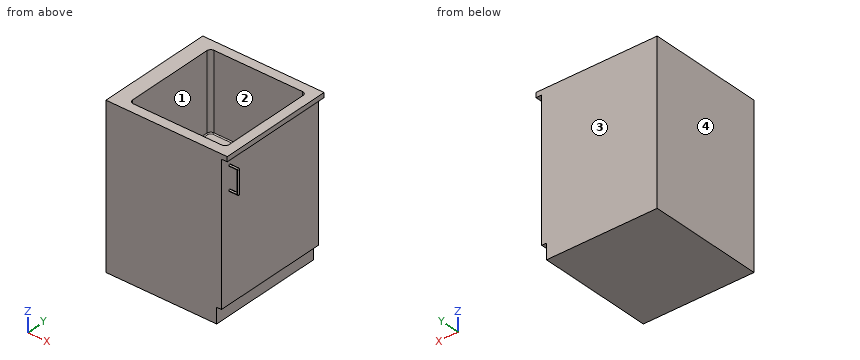
```python
from build123d import *

# Parameters (mm, degrees)
F0_W        = 600
F0_H        = 600
F1_DEPTH    = 800
F2_W        = 600
F2_H        = 80
F3_DEPTH    = 25
F5_DEPTH    = 50
F6_T1_DEPTH = 120
F6_T4_ANGLE = 180
F6_T6_ANGLE = 180
F7_W        = 40
F7_H        = 110
F8_DEPTH    = 25
F9_R        = 4.99999
F10_W       = 630
F10_H       = 600
F11_DEPTH   = 25
F13_DEPTH   = 400
F14_R       = 5
F16_D       = 50
F16_DEPTH   = 40
F16_TIP     = 15.0215154757


# Not quite as in the source:
# - a fillet or chamfer that OpenCascade refuses, or shapes differently, is made with other operations: its cross-section is extruded or revolved along the edge and cut away or added
# - a fillet or chamfer is up to 0.001 mm smaller than in the source, because OpenCascade refuses the exact size


with BuildPart() as f1:
    # F0 (on Top) → F1 (new body)
    with BuildSketch(Plane.XY):
        Rectangle(F0_W, F0_H)
    extrude(amount=F1_DEPTH)

    # F2 (on face) → F3 (cut)
    with BuildSketch(Plane.YZ.offset(300)):
        with Locations((0, 40)):
            Rectangle(F2_W, F2_H)
    extrude(amount=-F3_DEPTH, mode=Mode.SUBTRACT)

    # F4 (on face) → F5 (join)
    with BuildSketch(Plane.YZ.offset(300)):
        with BuildLine():
            ThreePointArc((-248.5795542598, 750), (-252.1150881657, 748.5355339059), (-253.5795542598, 745))
            Line((-253.5795542598, 745), (-253.5795542598, 625))
            ThreePointArc((-253.5795542598, 625), (-252.1150881657, 621.4644660941), (-248.5795542598, 620))
            ThreePointArc((-248.5795542598, 620), (-245.0440203538, 621.4644660941), (-243.5795542598, 625))
            Line((-243.5795542598, 625), (-243.5795542598, 745))
            ThreePointArc((-243.5795542598, 745), (-245.0440203538, 748.5355339059), (-248.5795542598, 750))
        make_face()
    extrude(amount=F5_DEPTH)

    # F6: fillet of radius 5 on 4 edges, made by hand

    # F6_s2 → F6_t1 (cut)
    with BuildSketch(Plane.XY.offset(625)):
        with BuildLine():
            ThreePointArc((345, -253.5795542598), (348.5355339059, -252.1150881657), (350, -248.5795542598))
            Line((350, -248.5795542598), (350, -253.5795542598))
            Line((350, -253.5795542598), (345, -253.5795542598))
        make_face()
        with BuildLine():
            ThreePointArc((345, -243.5795542598), (348.5355339059, -245.0440203538), (350, -248.5795542598))
            Line((350, -248.5795542598), (350, -243.5795542598))
            Line((350, -243.5795542598), (345, -243.5795542598))
        make_face()
    extrude(amount=F6_T1_DEPTH, mode=Mode.SUBTRACT)

    # F6_s3 → F6_t4 (revolve, cut)
    with BuildSketch(Plane.XY.offset(745)):
        with BuildLine():
            ThreePointArc((345, -253.5795542598), (348.5355339059, -252.1150881657), (350, -248.5795542598))
            Line((350, -248.5795542598), (350, -253.5795542598))
            Line((350, -253.5795542598), (345, -253.5795542598))
        make_face()
    revolve(axis=Axis((350, -248.5795542598, 745), (-1, 0, 0)), revolution_arc=F6_T4_ANGLE, mode=Mode.SUBTRACT)

    # F6_s5 → F6_t6 (revolve, cut)
    with BuildSketch(Plane.XY.offset(625)):
        with BuildLine():
            ThreePointArc((345, -243.5795542598), (348.5355339059, -245.0440203538), (350, -248.5795542598))
            Line((350, -248.5795542598), (350, -243.5795542598))
            Line((350, -243.5795542598), (345, -243.5795542598))
        make_face()
    revolve(axis=Axis((350, -248.5795542598, 625), (-1, 0, 0)), revolution_arc=F6_T6_ANGLE, mode=Mode.SUBTRACT)

    # F7 (on face) → F8 (cut)
    with BuildSketch(Plane(origin=(0, -243.5795542598, 0), x_dir=(-1, 0, 0), z_dir=(0, 1, 0))):
        with Locations((-320, 685)):
            Rectangle(F7_W, F7_H)
    extrude(amount=-F8_DEPTH, mode=Mode.SUBTRACT)

    # F9 (radius 5 in the source; OpenCascade refuses exactly that, so slightly less here)
    f9_edges = [f1.edges().sort_by_distance(p)[0] for p in [
        (320, -243.579554, 740),
        (340, -243.579554, 685),
        (320, -243.579554, 630),
        (320, -253.579554, 740),
        (340, -253.579554, 685),
        (320, -253.579554, 630),
    ]]
    fillet(f9_edges, radius=F9_R)

    # F10 (on face) → F11 (join)
    with BuildSketch(Plane.XY.offset(800)):
        with Locations((15, 0)):
            Rectangle(F10_W, F10_H)
    extrude(amount=F11_DEPTH)

    # F12 (on face) → F13 (cut)
    with BuildSketch(Plane.XY.offset(825)):
        with BuildLine():
            Line((-200, -250), (260, -250))
            ThreePointArc((260, -250), (274.1421356237, -244.1421356237), (280, -230))
            Line((280, -230), (280, 230))
            ThreePointArc((280, 230), (274.1421356237, 244.1421356237), (260, 250))
            Line((260, 250), (-200, 250))
            ThreePointArc((-200, 250), (-214.1421356237, 244.1421356237), (-220, 230))
            Line((-220, 230), (-220, -230))
            ThreePointArc((-220, -230), (-214.1421356237, -244.1421356237), (-200, -250))
        make_face()
    extrude(amount=-F13_DEPTH, mode=Mode.SUBTRACT)

    # F14
    f14_edges = [f1.edges().sort_by_distance(p)[0] for p in [
        (30, 250, 425),
        (-214.142136, 244.142136, 425),
        (-220, 0, 425),
        (30, -250, 425),
        (274.142136, -244.142136, 425),
        (280, 0, 425),
        (274.142136, 244.142136, 425),
        (-214.142136, -244.142136, 425),
    ]]
    fillet(f14_edges, radius=F14_R)

    # F16
    with Locations(Plane.XY.offset(425)):
        with Locations((-127.0953565836, 0)):
            Hole(F16_D / 2, depth=F16_DEPTH)
            with Locations((0, 0, -(F16_DEPTH + F16_TIP / 2))):  # 118° drill point
                Cone(0, F16_D / 2, F16_TIP, mode=Mode.SUBTRACT)


solid = f1.part
```
CAD build for the part. Positions are in the model's coordinates, mm. Face numbers are marked on the shaded views. Round coordinates to 2 decimals unless told otherwise and drop trailing zeros. Loops run counter-clockwise (first coordinate to the right, second up) from the corner with the lowest first, then second, coordinate; pieces in that order, holes last. Notation, with made-up numbers: M 11,70.5 L 44,70.5 A17 ccw 44,100.5 Z; hole C 62.25,76.5 d2. An arc over 180 degrees is marked long. Use a Markdown table: item, result. Add a question column.
(1) Cut at C-C (x = 50.5). Give the cut face in (y, z).
(2) Flat gauge pins, fed straight in: pin 1 (9 mm diameter, centred on x = 316.5, y = 117, fed in from -Z); pin 2 (6 mm diameter, centred on y = 89.5, z = 170.5, fed in from +X); pin 3 (7.5 mm diameter, centred on x = 287, y = -23, fed in from -Z). Where does each tip first touch, or does it go through?
(3) Drill centre lines: line 1 (X direction, y = 0, z = 417); line 2 (Y direction, x = 48, z = 590.5); line 3 (X direction, y = -41, z = 776.5). Where is each one in solid material? Low to high.
(4) Cut at A-A (y = -73.5). Give the cut face in (x, z), and give its area (3 significant figures).
(5) Cut at D-D (z = 56). Give the cut face in (x, y), and give its area (3 significant figures).
(6) Cut at B-B (z = 552). Give the cut face in (x, y), and give its area (3 significant figures).
(7) Pull direction X, two halves, no side cores. Call the marked faces 1, 2, 3 and 4: +X half, -X half, draft (parallel to the pull), parting line (faces both ways), or undercut.
Geometry says:
| question | item | result |
|---|---|---|
| 1 | outline | M -300,0 L 300,0 L 300,825 L 250,825 L 250,430 A5 cw 245,425 L -245,425 A5 cw -250,430 L -250,825 L -300,825 Z |
| 2 | pin 1 | stops at z = 800 |
| 2 | pin 2 | stops at x = 300 |
| 2 | pin 3 | stops at z = 80 |
| 3 | line 1 | x = -300 to -152.1, -102.1 to 300 |
| 3 | line 2 | y = -300 to -250, 250 to 300 |
| 3 | line 3 | x = -300 to -220, 280 to 300 |
| 4 | outline | M -300,0 L 275,0 L 275,80 L 300,80 L 300,800 L 330,800 L 330,825 L 280,825 L 280,430 A5 cw 275,425 L -215,425 A5 cw -220,430 L -220,825 L -300,825 Z |
| 4 | area | 294,000 mm² |
| 5 | outline | M -300,-300 L 275,-300 L 275,300 L -300,300 Z |
| 5 | area | 345,000 mm² |
| 6 | outline | M -300,-300 L 300,-300 L 300,300 L -300,300 Z; hole M -220,-230 A20 ccw -200,-250 L 260,-250 A20 ccw 280,-230 L 280,230 A20 ccw 260,250 L -200,250 A20 ccw -220,230 Z |
| 6 | area | 110,000 mm² |
| 7 | face 1 | undercut |
| 7 | face 2 | undercut |
| 7 | face 3 | draft |
| 7 | face 4 | -X half |
